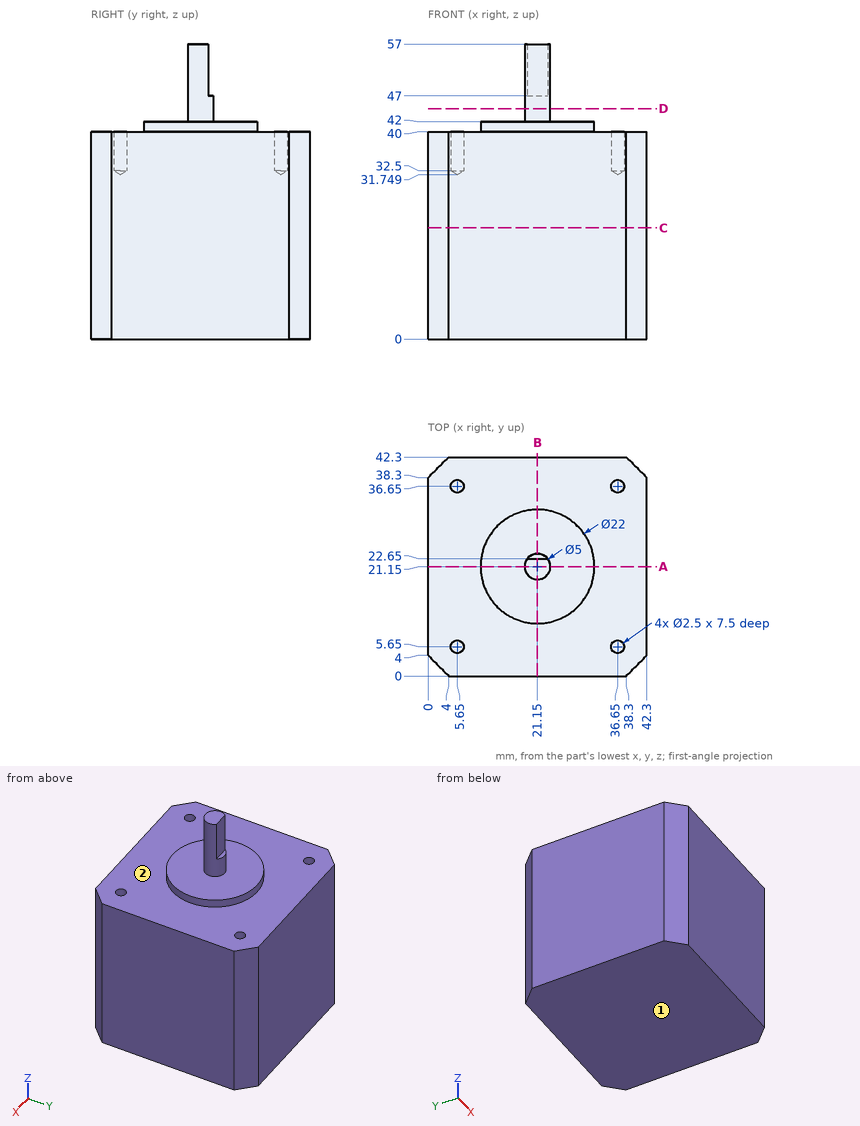
Here's the drawing with two shaded views (mm, measured from the low corner). I have some questions. A direction names the side the tool comes from. Give positions to 0.01 mm unless a question says otherwise; leave off trailing zeros. Loops run counter-clockwise (first coordinate to the right, second up) from the corner with the lowest first, then second, coordinate; pieces in that order, holes last. Notation, with made-up numbers: M 9.25,-26.5 L 59.25,-26.5 A14 cw 59.25,-19.5 Z; hole C -28,-2 d9. An arc over 180 degrees is marked long. One line per item, written item: value. Start each with the question number.
1) If we section it at B-B, the plane x = 21.15: Write out the boundary of the cut face in (y, z), and give its area (3 significant figures).
2) If I drill on line 1 (Y direction, x = 5.65, z = 36.5); line 2 (Y direction, x = 5, z = 35), over which ranges is the centre line in solid material (lowest first)? Write a range as [from, to].
3) If we section it at A-A, the plane y = 21.15: Write out the boundary of the cut face in (x, z).
4) If we section it at C-C, the plane z = 21.5: Write out the boundary of the cut face in (x, y), and give its area (3 significant figures).
5) I'm going to push flat-ended pins straight in: pin 1 (1.5 mm diameter, centred on x = 27.5, y = 32.5, fed in from -Z); pin 2 (3 mm diameter, centred on x = 21.5, z = 53, fed in from +Y); pin 3 (3 mm diameter, centred on x = 5.65, y = 36.65, fed in from +Z); pin 4 (10 mm diameter, centred on x = 24, y = 32.5, fed in from +Z). Where does each tip first touch, or does it pass through?
6) If we section it at D-D, the plane z = 44.5: Write out the boundary of the cut face in (x, y).
7) On a 3-axis mill with a long thin cutter (end or side, diameter ignored), from which of +Z, -Z, +X, -X, +Y, -Y can I reach the whole of each face in a straight line? I mean the marked faces 1 and 2. Say none if no direction works.
Completed:
1. outline: M 0,0 L 42.3,0 L 42.3,40 L 32.15,40 L 32.15,42 L 23.65,42 L 23.65,47 L 22.65,47 L 22.65,57 L 18.65,57 L 18.65,42 L 10.15,42 L 10.15,40 L 0,40 Z
1. area: 1,800 mm^2
2. line 1: y = [0, 4.4], [6.9, 35.4], [37.9, 42.3]
2. line 2: y = [0, 4.58], [6.72, 35.58], [37.72, 42.3]
3. outline: M 0,0 L 42.3,0 L 42.3,40 L 32.15,40 L 32.15,42 L 23.65,42 L 23.65,57 L 18.65,57 L 18.65,42 L 10.15,42 L 10.15,40 L 0,40 Z
4. outline: M 0,4 L 4,0 L 38.3,0 L 42.3,4 L 42.3,38.3 L 38.3,42.3 L 4,42.3 L 0,38.3 Z
4. area: 1,760 mm^2
5. pin 1: stops at z = 0
5. pin 2: stops at y = 22.65
5. pin 3: stops at z = 40
5. pin 4: stops at z = 42
6. outline: C 21.15,21.15 d5
7. face 1: -Z, +X, -X, +Y, -Y
7. face 2: +Z
